Input: part model. Units: mm. Frame: model coordinates. A direction names the side the tool comes from. Give positions to 0.01 mm unless a question says otherwise; leave off trailing zeros. Write each loop counter-clockwise with the first axis right and the second up, starting at its lowest first coordinate (ties: lowest second). Pieces come first, ordered by that corner, then holes.
```python
from build123d import *

# Parameters (mm, degrees)
SALIENTE_EXTRUIR1_DEPTH = 3
CROQUIS3_R              = 1
CROQUIS3_W              = 10
CROQUIS3_H              = 3
CROQUIS3_W_2            = 3
CROQUIS3_H_2            = 10
CORTAR_EXTRUIR1_DEPTH   = 4
CROQUIS4_R              = 1.5
CORTAR_EXTRUIR2_DEPTH   = 4
CROQUIS5_R              = 1.5
CORTAR_EXTRUIR3_DEPTH   = 4


with BuildPart() as part:
    # Croquis1 → Saliente-Extruir1 (new body)
    with BuildSketch(Plane(origin=(0, 0, 0), x_dir=(1, 0, 0), z_dir=(0, 1, 0))):
        Polygon((-47.5, 0), (-23.75, -41.13620668), (23.75, -41.13620668), (47.5, 0), (23.75, 41.13620668), (-23.75, 41.13620668), align=None)
    extrude(amount=SALIENTE_EXTRUIR1_DEPTH)

    # Croquis3 → Cortar-Extruir1 (cut, through all)
    with BuildSketch(Plane(origin=(0, 3, 0), x_dir=(1, 0, 0), z_dir=(0, 1, 0))):
        with Locations((-21.177619762, 19.723456661)):
            Circle(CROQUIS3_R)
        with Locations((18.822380238, 19.723456661)):
            Circle(CROQUIS3_R)
        with Locations((18.822380238, -18.276543339)):
            Circle(CROQUIS3_R)
        with Locations((-21.177619762, -18.276543339)):
            Circle(CROQUIS3_R)
        with Locations((-1.177619762, 19.723456661)):
            Rectangle(CROQUIS3_W, CROQUIS3_H)
        with Locations((35.322380238, 0.723456661)):
            Rectangle(CROQUIS3_W_2, CROQUIS3_H_2)
        with Locations((-1.177619762, -18.276543339)):
            Rectangle(CROQUIS3_W, CROQUIS3_H)
        with Locations((-37.677619762, 0.723456661)):
            Rectangle(CROQUIS3_W_2, CROQUIS3_H_2)
    extrude(amount=-CORTAR_EXTRUIR1_DEPTH, mode=Mode.SUBTRACT)

    # Croquis4 → Cortar-Extruir2 (cut, through all)
    with BuildSketch(Plane(origin=(0, 3, 0), x_dir=(1, 0, 0), z_dir=(0, 1, 0))):
        with Locations((20.005, -25.03)):
            Circle(CROQUIS4_R)
        with Locations((20.005, 25.03)):
            Circle(CROQUIS4_R)
        with Locations((-20.005, 25.03)):
            Circle(CROQUIS4_R)
        with Locations((-20.005, -25.03)):
            Circle(CROQUIS4_R)
    extrude(amount=-CORTAR_EXTRUIR2_DEPTH, mode=Mode.SUBTRACT)

    # Croquis5 → Cortar-Extruir3 (cut, through all)
    with BuildSketch(Plane(origin=(0, 3, 0), x_dir=(1, 0, 0), z_dir=(0, 1, 0))):
        with Locations((30, 17.5)):
            Circle(CROQUIS5_R)
        with Locations((30, -17.5)):
            Circle(CROQUIS5_R)
        with Locations((-30, -17.5)):
            Circle(CROQUIS5_R)
        with Locations((-30, 17.5)):
            Circle(CROQUIS5_R)
    extrude(amount=-CORTAR_EXTRUIR3_DEPTH, mode=Mode.SUBTRACT)


solid = part.part
```
Q1. Material intervals for line 1 along Z through (x, y) = (-1, 2.3); line 2 along Z through (x, y) = (30, 1.5); line 3 along X through (y, z) = (1.2, -25.03) (3 decimals), sorted ascending.
Q2. Section D-D, the plane z = -7.5. Return the cut outline in (x, y), then the cut area to 3 significant figures.
Q3. Pin query (flat end, axial travel): pin 1 (1.8 mm diameter, centred on x = 18.82, z = 18.28, fed in from +Y); pin 2 (5 mm diameter, centred on x = 20.005, z = 25.03, fed in from -Y); pin 3 (1.5 mm diameter, centred on y = 2, z = -1.5, fed in from +X); pin 4 (1.5 mm diameter, centred on y = 1, z = 3.5, fed in from +X). Return the tip coordinate at first contact, or that it passes through.
Q4. Section B-B, the plane z = 25.03. Return the cut outline in (x, y) (3 decimals).
Q5. Section A-A, the plane x = 2. Return the cut outline in (y, z), then the cut area to 3 significant figures.
Q6. Mould query, pull axis Z, two halves, no side actions, for faces 1 (the flat face through (-35.459, 1.479, -20.856)), 2 (the flat face through (0, 1, 41.136)), 3 (the flat face through (-38, 2, 4.277)), 4 (the flat face through (3.822, 2, -20)). Classes: +Z half, -Z half, draft (parallel to the pull), parting line (faces both ways), or undercut.
Q7. Section C-C, the plane y = 1.1. Give the number of separate pieces and of enclosed holes in the cut face, then the cut area to 3 significant figures.
Q8. Access query for faces 5 (the flat face through (-39.178, 2, -1)), 6 (the flat face through (35.459, 1.479, 20.856)). Directions: +Z, -Z, +X, -X, +Y, -Y. A direction counts if a zero-diameter tool reaches every point of the face in a straight line with its end or side. Return the directions, or none.
Solutions:
1. line 1: z = -41.14 to -21.22, -18.22 to 16.78, 19.78 to 41.14
1. line 2: z = -30.31 to -19, -16 to 16, 19 to 30.31
1. line 3: x = -33.049 to -21.505, -18.505 to 18.505, 21.505 to 33.049
2. outline: (-43.17, 0) - (43.17, 0) - (43.17, 3) - (-43.17, 3) - close
2. area: 259 mm2
3. pin 1: passes through
3. pin 2: stops at y = 0
3. pin 3: stops at x = 47.07
3. pin 4: stops at x = 45.91
4. outline: (-33.049, 0) - (-21.505, 0) - (-21.505, 3) - (-33.049, 3) - close; (-18.505, 0) - (18.505, 0) - (18.505, 3) - (-18.505, 3) - close; (21.505, 0) - (33.049, 0) - (33.049, 3) - (21.505, 3) - close
5. outline: (0, -41.14) - (3, -41.14) - (3, -21.22) - (0, -21.22) - close; (0, -18.22) - (3, -18.22) - (3, 16.78) - (0, 16.78) - close; (0, 19.78) - (3, 19.78) - (3, 41.14) - (0, 41.14) - close
5. area: 229 mm2
6. face 1: -Z half
6. face 2: +Z half
6. face 3: undercut
6. face 4: undercut
7. separate pieces: 1
7. enclosed holes: 16
7. area: 5,670 mm2
8. face 5: +Y, -Y
8. face 6: +Z, +X, +Y, -Y
